```python
from build123d import *

# Parameters (mm, degrees)
SKETCH1_W          = 12.7
SKETCH1_H          = 0.85725
SKETCH2_R          = 1.5
CUT_EXTRUDE1_DEPTH = 24.14921219


with BuildPart() as part:
    # Sketch1 → Revolve1 (revolve)
    with BuildSketch(Plane.XY, mode=Mode.PRIVATE) as revolve1_sk:
        with Locations((6.35, 3.603625)):
            Rectangle(SKETCH1_W, SKETCH1_H)
        Polygon((12.7, 4.03225), (12.7, 3.175), (14.605, 3.175), (14.605, 12.7), (12.7, 12.7), align=None)
        with Locations((-6.35, 3.603625)):
            Rectangle(SKETCH1_W, SKETCH1_H)
        Polygon((-14.605, 3.175), (-12.7, 3.175), (-12.7, 4.03225), (-12.7, 12.7), (-14.605, 12.7), align=None)
    revolve(revolve1_sk.sketch.rotate(Axis((-15.275524476, 0, 0), (1, 0, 0)), 90), axis=Axis((-15.275524476, 0, 0), (1, 0, 0)))

    # Sketch2 → Cut-Extrude1 (cut, through all)
    with BuildSketch(Plane(origin=(0, 0, 0), x_dir=(1, 0, 0), z_dir=(0, 1, 0))):
        with Locations(Location((0, 0, 0), (0, 0, 90))):
            Circle(SKETCH2_R)
    extrude(amount=CUT_EXTRUDE1_DEPTH, mode=Mode.SUBTRACT)


solid = part.part
```
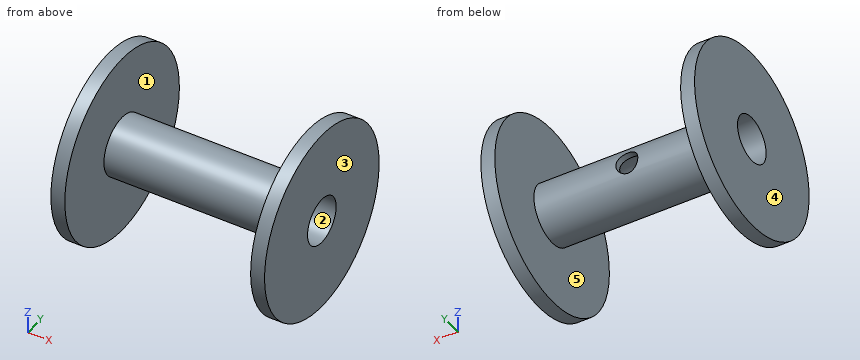
Design review of the part built by this model. Coordinates are the model's own, in mm. Face numbers are marked on the shaded views. A direction names the side the tool comes from. Coordinates: 2 decimals unless noted, no trailing zeros. Order: outer loops, then holes, each group sorted by start corner. A loop starts at its lowest first (then second) coordinate and runs counter-clockwise, first axis right, second up. Notation, with made-up numbers: M 40.25,67 L 86.25,67 A30 ccw 86.25,97 Z; hole C -27,25 d8. An arc over 180 degrees is marked long. Answer as a JSON object with one key per item and string values. Group by question number.
1) Mouldability with a two-part tool opening along X and no side actions: class the marked faces 3, 4 and 5 as pulls with the +X half, pulls with the -X half, needs draft (parallel to the pull), parting line crosses it, or undercut.
2) Wall thickness on L1, parallel to X at y = -9.75, z = -0.5 (3 decimals); L2, parallel to X at y = 3.7, z = 0 (3 decimals); L3, parallel to Y at x = -2.75, z = 0 (3 decimals): over which ranges is each line inside the solid? List them lowest first.
3) Add section D-D, the plane y = 8. Write out the cut boundary in (x, z) (3 decimals).
4) Tool access review of the marked faces 1 and 2: name each direction out of +Z, -Z, +X, -X, +Y, -Y from which nothing blocks a thin tool from reaching the whole face with its end or side.
5) Add section B-B, the plane y = 2. Write out the cut boundary in (x, z) (3 decimals), then the cut area to 3 significant figures.
6) For pin 1 (8 mm diameter, centred on x = 4.5, z = 1, fed in from -Y); pin 2 (5 mm diameter, centred on x = 7, z = -1.5, fed in from +Y); pin 3 (10 mm diameter, centred on x = -6.5, y = -4, fed in from -Z), all flat-tipped, find the tip position at first contact; note any pin that passes through.
7) Add section A-A, the plane z = 0. Write out the cut boundary in (x, y) (3 decimals).
Computed values:
{
 "1": {"face 3": "pulls with the +X half", "face 4": "pulls with the -X half", "face 5": "undercut"},
 "2": {"L1": "x = -14.605 to -12.7, 12.7 to 14.605", "L2": "x = -14.605 to -1.5, 1.5 to 14.605", "L3": "y = -4.032 to -3.175, 3.175 to 4.032"},
 "3": {"outline": "M -14.605,-9.864 L -12.7,-9.864 L -12.7,9.864 L -14.605,9.864 Z; M 12.7,-9.864 L 14.605,-9.864 L 14.605,9.864 L 12.7,9.864 Z"},
 "4": {"face 1": "none", "face 2": "+X, -X"},
 "5": {"outline": "M -14.605,-12.542 L -12.7,-12.542 L -12.7,-3.501 L 12.7,-3.501 L 12.7,-12.542 L 14.605,-12.542 L 14.605,-2.466 L -14.605,-2.466 Z; M -14.605,2.466 L 14.605,2.466 L 14.605,12.542 L 12.7,12.542 L 12.7,3.501 L -12.7,3.501 L -12.7,12.542 L -14.605,12.542 Z", "area": "129 mm^2"},
 "6": {"pin 1": "stops at y = -4.03", "pin 2": "stops at y = 4.03", "pin 3": "stops at z = -4.03"},
 "7": {"outline": "M -14.605,-12.7 L -12.7,-12.7 L -12.7,-4.032 L 12.7,-4.032 L 12.7,-12.7 L 14.605,-12.7 L 14.605,-3.175 L -14.605,-3.175 Z; M -14.605,3.175 L -1.5,3.175 L -1.5,4.032 L -12.7,4.032 L -12.7,12.7 L -14.605,12.7 Z; M 1.5,3.175 L 14.605,3.175 L 14.605,12.7 L 12.7,12.7 L 12.7,4.032 L 1.5,4.032 Z"}
}
